The model under review builds one solid part; all positions refer to its coordinate system, in mm. Give positions to 0.01 mm unless a question says otherwise; leave off trailing zeros. Order: outer loops, then holes, each group sorted by start corner. A loop starts at its lowest first (then second) coordinate and runs counter-clockwise, first axis right, second up. Notation, with made-up numbers: (23.25, 38.5) - (81.25, 38.5) arc R29 cw to (81.25, 66.5) - close; hole circle Ø2 at (55.25, -8.5). An arc over 180 degrees is marked (long way). Put each result on its own line as item: value.
```python
from build123d import *

# Parameters (mm, degrees)
SKETCH1_W               = 120
SKETCH1_H               = 80
BOSS_EXTRUDE1_DEPTH     = 6
CUT_EXTRUDE3_DEPTH      = 73.360210061
CUT_EXTRUDE3_DEPTH_BACK = 73.360210061
SKETCH2_R               = 3.5


with BuildPart() as part:
    # Sketch1 → Boss-Extrude1 (new body)
    with BuildSketch(Plane.XY):
        Rectangle(SKETCH1_W, SKETCH1_H)
    extrude(amount=BOSS_EXTRUDE1_DEPTH)

    # Sketch2 → Cut-Extrude3 (cut, two sides: drawn at the far end of the back side and taken through both)
    with BuildSketch(Plane.XY.offset(-CUT_EXTRUDE3_DEPTH_BACK)):
        Circle(SKETCH2_R)
    extrude(amount=CUT_EXTRUDE3_DEPTH + CUT_EXTRUDE3_DEPTH_BACK, mode=Mode.SUBTRACT)


solid = part.part
```
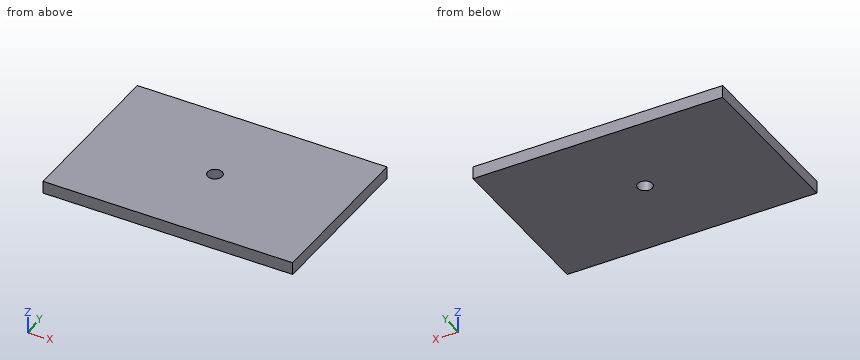
(1) Take a section at B-B, the plane x = 0. Write out the cut boundary in (y, z), then the cut area to 3 significant figures.
The answers:
outline: (-40, 0) - (-3.5, 0) - (-3.5, 6) - (-40, 6) - close; (3.5, 0) - (40, 0) - (40, 6) - (3.5, 6) - close
area: 438 mm^2
(2) Wall thickness on L1, parallel to Y at x = 0, z = 4.3; L2, parallel to X at y = 0, z = 4; L3, parallel to Y at x = -2, z = 4.55: over which ranges is each line inside the solid? List them lowest first.
The answers:
L1: -40 to -3.5, 3.5 to 40
L2: -60 to -3.5, 3.5 to 60
L3: -40 to -2.87, 2.87 to 40
(3) Take a section at A-A, the plane y = 0. Write out the cut boundary in (x, z).
The answers:
outline: (-60, 0) - (-3.5, 0) - (-3.5, 6) - (-60, 6) - close; (3.5, 0) - (60, 0) - (60, 6) - (3.5, 6) - close
